Verification items for the finished model (mm, model axes). A direction names the side the tool comes from. Coordinates: 2 decimals unless noted, no trailing zeros. Write each loop counter-clockwise with the first axis right and the second up, starting at its lowest first coordinate (ties: lowest second). Pieces come first, ordered by that corner, then holes. Notation, with made-up numbers: M 3.25,-24 L 26.25,-24 A17 ccw 26.25,5 Z; hole C -20,6 d5. An arc over 180 degrees is marked long. Answer in a Markdown table with one row per item.
Autodesk Fusion 360 part; units mm, degrees
sketch "Sketch1" plane through (0, 0, 0) normal (0, 0, 1) x (1, 0, 0)
  circle A0 centre (0, 0) radius 1.75
  circle A1 centre (18.5, 0) radius 1.75
  line L0 (-20, 7) -> (24.5, 7)
  line L1 (24.5, 7) -> (24.5, -7)
  line L2 (24.5, -7) -> (-20, -7)
  line L3 (-20, -7) -> (-20, 7)
  arc A2 (-20, -7) -> (-107.1054, -25.8531) centre (-20, -217.6501) ccw
  arc A3 (-20, -7) -> (-20, 7) centre (-20, 0) ccw
  arc A4 (-20, 7) -> (-112.8946, -13.106) centre (-20, -217.6501) ccw
  arc A5 (-112.8946, -13.106) -> (-107.1054, -25.8531) centre (-110, -19.4796) ccw
  arc A6 (-20, 0) -> (-110, -19.4796) centre (-20, -217.6501) ccw construction
  dimension "d1" = 3.5
  dimension "d2" = 3.5
  dimension "d3" = 18.5
  dimension "d4" = 6
  dimension "d5" = 7
  dimension "d6" = 7
  dimension "d7" = 20
extrude "Extrude1" add sketch "Sketch1" along normal blind 4 contours A0 | A1 | L3 A3 | L0 L1 L2 A3 | L3 A2 A4 A5
extrude "Extrude2" add sketch "Sketch1" along normal blind 19 contours L3 A2 A4 A5
extrude "Extrude3" add sketch "Sketch1" along normal blind 4 from surface at 15 contours A0 | A1 | L3 A3 | L0 L1 L2 A3 | L3 A2 A4 A5
extrude "Extrude4" cut sketch "Sketch1" along normal blind 35 contours A0
extrude "Extrude5" cut sketch "Sketch1" along normal blind 19 contours A1
fillet "Fillet1" radius 4 4 edges at (24.5, -7, 17) (24.5, -7, 2) (24.5, 7, 17) (24.5, 7, 2)
fillet "Fillet2" radius 1.5 16 edges at (-64.5612, -11.7672, 19) (0.25, -7, 19) (23.3284, -5.8284, 19) (24.5, 0, 19) (23.3284, 5.8284, 19) (0.25, 7, 19) (-67.5228, 1.916, 19) (-116.3735, -22.3741, 19) (-64.5612, -11.7672, 0) (0.25, -7, 0) (23.3284, -5.8284, 0) (24.5, 0, 0) (23.3284, 5.8284, 0) (0.25, 7, 0) (-67.5228, 1.916, 0) (-116.3735, -22.3741, 0)
1) Sectioned sample at C-C (z = 9.25). Record the cut outline in (x, y).
Response values:
| item | result |
|---|---|
| outline | M -112.89,-13.11 A7 ccw -107.11,-25.85 A210.65 cw -20,-7 L -20,7 A224.65 ccw Z |
2) Sectioned sample at A-A (x = 18.5). Record the cut outline in (y, z), then the cut area to 3 significant figures.
Response values:
| item | result |
|---|---|
| outline | M -7,1.5 A1.5 ccw -5.5,0 L -1.75,0 L -1.75,4 L -7,4 Z; M -7,15 L -1.75,15 L -1.75,19 L -5.5,19 A1.5 ccw -7,17.5 Z; M 1.75,0 L 5.5,0 A1.5 ccw 7,1.5 L 7,4 L 1.75,4 Z; M 1.75,15 L 7,15 L 7,17.5 A1.5 ccw 5.5,19 L 1.75,19 Z |
| area | 82.1 mm² |
3) Tool access check on faces 1 (the face through (24.5, 0, 3)), 2 (the face through (1, -7, 16)), 3 (the face through (2, 0, 15)). Record the directions out of +Z, -Z, +X, -X, +Y, -Y that give a thin tool (end or side, any length) a straight path to the whole face; none if there is none.
Response values:
| item | result |
|---|---|
| face 1 | +Z, -Z, +X, +Y, -Y |
| face 2 | +Z, -Z, +X, -Y |
| face 3 | +X, +Y, -Y |
4) Release check for a two-part mould opening along Y. For faces 4 (the face through (16.75, -0.08, 16.97)), 5 (the face through (23.297, -5.859, 2.768)), 6 (the face through (-20, 0, 9)), 7 (the face through (23.359, 5.797, 16.267)) record: +Y half, -Y half, draft (parallel to the pull), parting line (faces both ways), or undercut.
Response values:
| item | result |
|---|---|
| face 4 | undercut |
| face 5 | -Y half |
| face 6 | draft |
| face 7 | +Y half |
5) Sectioned sample at B-B (y = 0). Give the number of separate pieces and of enclosed holes in the cut face, then the cut area to 3 significant figures.
Response values:
| item | result |
|---|---|
| separate pieces | 5 |
| enclosed holes | 0 |
| area | 1,350 mm² |
6) Depth check by flat-ended pin: pin 1 (1.2 mm diameter, centred on x = 6.5, z = 15.5, fed in from -Y); pin 2 (3 mm diameter, centred on x = -41.5, z = 2.5, fed in from +Y); pin 3 (10 mm diameter, centred on x = -87, z = 9, fed in from -Y). Enter the tip coordinate at first touch or a pass-through.
Response values:
| item | result |
|---|---|
| pin 1 | stops at y = -7 |
| pin 2 | stops at y = 6.11 |
| pin 3 | stops at y = -19.69 |
7) Thickness scan on L1, parallel to Z at x = -7, y = 5; L2, parallel to Y at x = 0, z = 16.3; L3, parallel to Y at x = -105, z = 3.5. Record the ranges inside material, lowest first. Write a range as [from, to].
Response values:
| item | result |
|---|---|
| L1 | z = [0, 4], [15, 19] |
| L2 | y = [-7, -1.75], [1.75, 7] |
| L3 | y = [-24.91, -9.7] |
